For this review, take the finished solid that the model builds, in its own axes (mm). A direction names the side the tool comes from. Coordinates: 2 decimals unless noted, no trailing zeros. Loops run counter-clockwise (first coordinate to the right, second up) from the corner with the lowest first, then second, coordinate; pieces in that order, holes last. Notation, with made-up numbers: (-14.75, 78) - (42.25, 78) arc R22 cw to (42.25, 100) - close; hole circle Ø8 at (29.5, 48.25). An arc over 180 degrees is marked (long way). Answer as a JSON object with one key per item and string values. Group by question number.
Item 1: We need section B-B (x = 0). Give the boundary of the cut face in (y, z), then the cut area to 3 significant figures.
Item 2: We need section C-C (y = -24). Give the boundary of the cut face in (x, z).
Item 3: We need section A-A (y = 24.8). Give the boundary of the cut face in (x, z).
Item 4: Tool access review of faces 1 (the cylindrical face through (2.045, 78.025, -92.978)), 2 (the flat face through (99, 34.8, -10)), 3 (the flat face through (26, 64.8, -97)), 4 (the flat face through (100.933, -35, -26)): name each direction out of +Z, -Z, +X, -X, +Y, -Y from which nothing blocks a thin tool from reaching the whole face with its end or side.
Item 5: Mouldability with a two-part tool opening along X and no side actions: class faces 5 (the flat face through (104, 23, -20)), 6 (the cylindrical face through (25.34, 72.4, -94.15)), 7 (the cylindrical face through (112, 25, -10)) as released by +X, released by -X, zero draft, split by the parting line, or undercut.
Item 6: To check wall thickness, follow line 1 (Y direction, x = 102, z = -14.5); line 2 (X direction, y = 25.5, z = -8); line 3 (Y direction, x = -102, z = -13.25). State the ranges of each line that lie inside material, in increasing order.
Item 7: Clearance check with flat-ended pins moving along their axes: pin 1 (1.6 mm diameter, centred on y = 33.5, z = 1.5, fed in from +X); pin 2 (8.5 mm diameter, centred on x = -102, y = 24.8, fed in from -Z); pin 3 (15 mm diameter, centred on x = 98.5, y = 26, fed in from +Z); pin 4 (5.5 mm diameter, centred on x = -90.93, z = -52.5, fed in from +Y). State where each tip first meets the part, or that it passes through.
from build123d import *

# Parameters (mm, degrees)
REVOLU_O2_ANGLE             = 180
ESBO_O4_R                   = 10
RESSALTO_EXTRUS_O1_DEPTH    = 35
RESSALTO_EXTRUS_O10_DEPTH   = 10
ESBO_O8_R                   = 3.5
CORTE_EXTRUS_O2_DEPTH       = 20
PADR_OCIRCULAR1_COUNT       = 6
ESBO_O6_R                   = 2.5
CORTE_EXTRUS_O1_DEPTH       = 15
ESBO_O9_R                   = 1.25
CORTE_EXTRUS_O3_DEPTH       = 6
ESBO_O10_W                  = 2.2
ESBO_O10_H                  = 116.4
CORTE_EXTRUS_O4_DEPTH       = 3.5
ESBO_O11_W                  = 2
ESBO_O11_H                  = 114.9
RESSALTO_EXTRUS_O5_DEPTH    = 2
ESBO_O12_R                  = 3.25
RESSALTO_EXTRUS_O6_DEPTH    = 20
ESBO_O13_R                  = 2.5
RESSALTO_EXTRUS_O7_DEPTH    = 20
ESBO_O16_R                  = 93
CORTE_EXTRUS_O6_DEPTH       = 10
ESBO_O25_R                  = 60.842408243
CORTE_EXTRUS_O10_DEPTH      = 44.15
CORTE_EXTRUS_O10_DEPTH_BACK = 77.85


with BuildPart() as part:
    # Esbo_o3 → Revolu_o2 (revolve)
    with BuildSketch(Plane.XY):
        with BuildLine():
            Line((97.5, 79.8), (97.5, 11.304491341))
            Line((97.5, 11.304491341), (97.5, 0))
            Line((97.5, 0), (97.5, -40.2))
            Line((97.5, -40.2), (79.5, -40.2))
            Line((79.5, -40.2), (79.5, 0))
            Line((79.5, 0), (60.342408243, 0))
            Line((60.342408243, 0), (60.342408243, 2.95))
            Line((60.342408243, 2.95), (52, 2.95))
            Line((52, 2.95), (44, 10.95))
            Line((44, 10.95), (31, 10.95))
            Line((31, 10.95), (31, 13.7))
            Line((31, 13.7), (22.6, 13.7))
            Line((22.6, 13.7), (22.6, 17))
            Line((22.6, 17), (19.3, 17))
            Line((19.3, 17), (19.3, 17.7))
            Line((19.3, 17.7), (15.3, 17.7))
            Line((15.3, 17.7), (15.3, 21.05))
            Line((15.3, 21.05), (19.3, 21.05))
            Line((19.3, 21.05), (19.3, 21.2))
            Line((19.3, 21.2), (27.626549127, 25.96))
            Line((27.626549127, 25.96), (31.3, 25.96))
            Line((31.3, 25.96), (31.3, 43.96))
            Line((31.3, 43.96), (32.3, 44.96))
            Line((32.3, 44.96), (38.8, 44.96))
            Line((38.8, 44.96), (38.8, 26.9))
            Line((38.8, 26.9), (55.5, 10.2))
            Line((55.5, 10.2), (83.5, 10.2))
            ThreePointArc((83.5, 10.2), (86.328427125, 11.371572875), (87.5, 14.2))
            Line((87.5, 14.2), (87.5, 76.2))
            Line((87.5, 76.2), (93, 76.2))
            Line((93, 76.2), (93, 79.8))
            Line((93, 79.8), (97.5, 79.8))
        make_face()
    revolve(axis=Axis((0, -3.322055656, 0), (0, 1, 0)), revolution_arc=REVOLU_O2_ANGLE)

    # Esbo_o4 → Ressalto-extrus_o1 (add)
    with BuildSketch(Plane(origin=(0, 79.8, 0), x_dir=(1, 0, 0), z_dir=(0, 1, 0))):
        with Locations((25.881656302, 96.591656302)):
            Circle(ESBO_O4_R)
        with Locations((-96.591656302, 25.881656302)):
            Circle(ESBO_O4_R)
    extrude(amount=-RESSALTO_EXTRUS_O1_DEPTH)

    # Esbo_o23 → Ressalto-extrus_o10 (add)
    with BuildSketch(Plane.XZ.offset(40.2)):
        with BuildLine():
            Line((95.932667397, -61.160254038), (5, -113.660254038))
            ThreePointArc((5, -113.660254038), (0, -115), (-5, -113.660254038))
            Line((-5, -113.660254038), (-95.932667397, -61.160254038))
            ThreePointArc((-95.932667397, -61.160254038), (-99.592921435, -57.5), (-100.932667397, -52.5))
            Line((-100.932667397, -52.5), (-100.932667397, 0))
            Line((-100.932667397, 0), (-96.380584002, 0))
            ThreePointArc((-96.380584002, 0), (0, -96.380584002), (96.380584002, 0))
            Line((96.380584002, 0), (100.932667397, 0))
            Line((100.932667397, 0), (100.932667397, -52.5))
            ThreePointArc((100.932667397, -52.5), (99.592921435, -57.5), (95.932667397, -61.160254038))
        make_face()
    extrude(amount=-RESSALTO_EXTRUS_O10_DEPTH)

    # Esbo_o8 → Corte-extrus_o2 (cut)
    with BuildSketch(Plane.XZ.offset(40.2)):
        with Locations((0, -105)):
            Circle(ESBO_O8_R)
    corte_extrus_o2 = extrude(amount=-CORTE_EXTRUS_O2_DEPTH, mode=Mode.SUBTRACT)

    # Padr_oCircular1: Corte-extrus_o2 ×6 about axis
    padr_ocircular1_axis = Axis((0, 0, 0), (0, 1, 0))
    for i in range(1, PADR_OCIRCULAR1_COUNT):
        add(corte_extrus_o2.rotate(padr_ocircular1_axis, i * 360 / PADR_OCIRCULAR1_COUNT), mode=Mode.SUBTRACT)

    # Esbo_o6 → Corte-extrus_o1 (cut)
    with BuildSketch(Plane(origin=(0, 79.8, 0), x_dir=(1, 0, 0), z_dir=(0, 1, 0))):
        with Locations((25.881656302, 96.591656302)):
            Circle(ESBO_O6_R)
        with Locations((-96.591656302, 25.881656302)):
            Circle(ESBO_O6_R)
    extrude(amount=-CORTE_EXTRUS_O1_DEPTH, mode=Mode.SUBTRACT)

    # Esbo_o9 → Corte-extrus_o3 (cut)
    with BuildSketch(Plane.XZ.offset(-13.7)):
        with Locations((18.738329701, -18.738329701)):
            Circle(ESBO_O9_R)
        with Locations((-18.738329701, -18.738329701)):
            Circle(ESBO_O9_R)
        with Locations((-18.738329701, 18.738329701)):
            Circle(ESBO_O9_R)
        with Locations((18.738329701, 18.738329701)):
            Circle(ESBO_O9_R)
    extrude(amount=-CORTE_EXTRUS_O3_DEPTH, mode=Mode.SUBTRACT)

    # Esbo_o10 → Corte-extrus_o4 (cut)
    with BuildSketch(Plane.XY):
        with Locations((92, 18)):
            Rectangle(ESBO_O10_W, ESBO_O10_H)
    extrude(amount=-CORTE_EXTRUS_O4_DEPTH, mode=Mode.SUBTRACT)

    # Esbo_o11 → Ressalto-extrus_o5 (add)
    with BuildSketch(Plane.XY):
        with Locations((-92, 18.75)):
            Rectangle(ESBO_O11_W, ESBO_O11_H)
    extrude(amount=RESSALTO_EXTRUS_O5_DEPTH)

    # Esbo_o12 → Ressalto-extrus_o6 (add)
    with BuildSketch(Plane.XY):
        with BuildLine():
            Line((-102, 34.8), (-87.5, 34.8))
            Line((-87.5, 34.8), (-87.5, 14.8))
            Line((-87.5, 14.8), (-102, 14.8))
            ThreePointArc((-102, 14.8), (-112, 24.8), (-102, 34.8))
        make_face()
        with Locations((-102, 24.8)):
            Circle(ESBO_O12_R, mode=Mode.SUBTRACT)
    extrude(amount=-RESSALTO_EXTRUS_O6_DEPTH)

    # Esbo_o13 → Ressalto-extrus_o7 (add)
    with BuildSketch(Plane.XY):
        with BuildLine():
            Line((102, 34.8), (93.1, 34.8))
            Line((93.1, 34.8), (93.1, 14.8))
            Line((93.1, 14.8), (102, 14.8))
            ThreePointArc((102, 14.8), (112, 24.8), (102, 34.8))
        make_face()
        with Locations((102, 24.8)):
            Circle(ESBO_O13_R, mode=Mode.SUBTRACT)
    extrude(amount=-RESSALTO_EXTRUS_O7_DEPTH)

    # Esbo_o16 → Corte-extrus_o6 (cut)
    with BuildSketch(Plane(origin=(0, 76.2, 0), x_dir=(1, 0, 0), z_dir=(0, 1, 0))):
        Circle(ESBO_O16_R)
    extrude(amount=CORTE_EXTRUS_O6_DEPTH, mode=Mode.SUBTRACT)

    # Esbo_o25 → Corte-extrus_o10 (cut, two sides)
    with BuildSketch(Plane.XZ.offset(-2.95)) as corte_extrus_o10_sk:
        Circle(ESBO_O25_R)
    extrude(amount=CORTE_EXTRUS_O10_DEPTH, mode=Mode.SUBTRACT)
    extrude(corte_extrus_o10_sk.sketch, amount=-CORTE_EXTRUS_O10_DEPTH_BACK, mode=Mode.SUBTRACT)


solid = part.part
Check sheet entries:
{
 "1": {"outline": "(-40.2, -115) - (-30.2, -115) - (-30.2, -108.5) - (-40.2, -108.5) - close; (-40.2, -101.5) - (-30.2, -101.5) - (-30.2, -97.5) - (79.8, -97.5) - (79.8, -93) - (76.2, -93) - (76.2, -87.5) - (14.2, -87.5) arc R4 cw to (10.2, -83.5) - (10.2, -60.84) - (0, -60.84) - (0, -79.5) - (-40.2, -79.5) - close", "area": "1,880 mm2"},
 "2": {"outline": "(-97.5, 0) arc R97.5 ccw to (97.5, 0) - (93.1, 0) - (93.1, -3.5) - (90.9, -3.5) - (90.9, 0) - (79.5, 0) arc R79.5 cw to (-79.5, 0) - (-91, 0) - (-91, 2) - (-93, 2) - (-93, 0) - close"},
 "3": {"outline": "(-112, -20) - (-105.25, -20) - (-105.25, 0) - (-112, 0) - close; (-98.75, -20) - (-95.43, -20) arc R97.5 ccw to (95.43, -20) - (99.5, -20) - (99.5, 0) - (93.1, 0) - (93.1, -3.5) - (90.9, -3.5) - (90.9, 0) - (87.5, 0) arc R87.5 cw to (-87.5, 0) - (-91, 0) - (-91, 2) - (-93, 2) - (-93, 0) - (-98.75, 0) - close; (104.5, -20) - (112, -20) - (112, 0) - (104.5, 0) - close"},
 "4": {"face 1": "+Z, +Y", "face 2": "-Z, +X, +Y", "face 3": "+Y", "face 4": "+Z, -Z, +X, -Y"},
 "5": {"face 5": "zero draft", "face 6": "undercut", "face 7": "released by +X"},
 "6": {"line 1": "y = 14.8 to 22.3, 27.3 to 34.8", "line 2": "x = -111.98 to -105.17, -98.83 to -87.13, 87.13 to 99.6, 104.4 to 111.98", "line 3": "y = 14.8 to 21.55, 28.05 to 34.8"},
 "7": {"pin 1": "stops at x = -91", "pin 2": "stops at z = -20", "pin 3": "stops at z = 0", "pin 4": "passes through"}
}
